Source: CAD feature listing. Evaluate the final solid. Frame: model axes, mm. A direction names the side the tool comes from. Coordinates: 2 decimals unless noted, no trailing zeros. Write each loop counter-clockwise with the first axis right and the second up, starting at its lowest first coordinate (ties: lowest second). Pieces come first, ordered by that corner, then holes. Notation, with made-up numbers: (54, 30) - (73, 30) arc R27 ccw to (73, 51) - close; hole circle Ø11 at (70.25, 13.5). An arc over 180 degrees is marked (long way). One line per question, with ' | ' between items. Start each with the question number.
Q1. Draft query along Y for faces 1 (the face through (71, -23.57, 14.2)), 2 (the face through (-72.15, -56.99, 20.28)), 3 (the face through (0.91, 57.15, 46.99)), 4 (the face through (-18.07, -0.28, 31.5)). Return one class per face: +Y half, -Y half, draft (parallel to the pull), parting line (faces both ways), or undercut.
Q2. Cut plane D-D, the plane y = 23. Return loops of the section in (x, z), plus the area to 3 significant figures.
Q3. Cut plane A-A, the plane y = 0. Return loops of the section in (x, z).
Q4. Cut plane B-B, the plane z = 35.5. Return loops of the section in (x, y), plus the area to 3 significant figures.
Q5. Line query: line 1 (Y direction, x = -43, z = 13.5); line 2 (Y direction, x = 54, z = 27); line 3 (Z direction, x = 37, y = 7). Output: solid intervals per line, ascending.
Q6. Cut plane C-C, the plane x = 5. Return loops of the section in (y, z).
Q7. Contact query for flat-ended pins moving along their axis: P1, Ø0.8, axis at x = 74.5, y = -1.5, coming from the +Z side; P2, Ø20, axis at x = 31, y = 6, coming from the -Z side. Output: stop coordinate, or through.
Q8. Access query for faces 5 (the face through (-72.15, 56.99, 20.28)), 6 (the face through (27, -24, 31)). Directions: +Z, -Z, +X, -X, +Y, -Y. A direction counts if a zero-diameter tool reaches every point of the face in a straight line with its end or side. Return the directions, or none.
```python
from build123d import *

# Parameters (mm, degrees)
F0_W     = 150
F0_H     = 120
F1_DEPTH = 50
F2_R     = 10
F3_W     = 92
F3_H     = 50
F4_DEPTH = 33
F5_R     = 5
F6_W     = 25
F6_H     = 10.0465611815
F7_DEPTH = 40
F9_DEPTH = 25


with BuildPart() as f1:
    # F0 (on Top) → F1 (new body)
    with BuildSketch(Plane.XY):
        Rectangle(F0_W, F0_H)
    extrude(amount=F1_DEPTH)

    # F2
    f2_edges = [f1.edges().sort_by_distance(p)[0] for p in [
        (0, -60, 50),
        (-75, 0, 50),
        (0, 60, 50),
        (75, 0, 50),
        (-75, -60, 25),
        (75, -60, 25),
        (75, 60, 25),
        (-75, 60, 25),
    ]]
    fillet(f2_edges, radius=F2_R)

    # F3 (on face) → F4 (cut)
    with BuildSketch(Plane(origin=(0, 0, 0), x_dir=(1, 0, 0), z_dir=(0, 0, -1))):
        with Locations((26.5, 0)):
            Rectangle(F3_W, F3_H)
    extrude(amount=-F4_DEPTH, mode=Mode.SUBTRACT)

    # F5
    f5_edges = [f1.edges().sort_by_distance(p)[0] for p in [
        (26.5, 25, 33),
        (72.5, 0, 33),
        (26.5, -25, 33),
        (-19.5, 0, 33),
        (-19.5, -25, 16.5),
        (72.5, -25, 16.5),
        (-19.5, 25, 16.5),
        (72.5, 25, 16.5),
    ]]
    fillet(f5_edges, radius=F5_R)

    # F6 (on face) → F7 (cut)
    with BuildSketch(Plane(origin=(0, 0, 0), x_dir=(1, 0, 0), z_dir=(0, 0, -1))):
        with Locations((-32, -14)):
            Rectangle(F6_W, F6_H)
    extrude(amount=-F7_DEPTH, mode=Mode.SUBTRACT)

    # F8 (on face) → F9 (cut)
    with BuildSketch(Plane.YZ.offset(75)):
        with BuildLine():
            Line((12, 18), (0, 18))
            ThreePointArc((0, 18), (1.7573593129, 13.7573593129), (6, 12))
            ThreePointArc((6, 12), (10.2426406871, 13.7573593129), (12, 18))
        make_face()
        with BuildLine():
            ThreePointArc((6, 24), (1.7573593129, 22.2426406871), (0, 18))
            Line((0, 18), (12, 18))
            ThreePointArc((12, 18), (10.2426406871, 22.2426406871), (6, 24))
        make_face()
        with BuildLine():
            ThreePointArc((-6, 24), (-1.7573593129, 22.2426406871), (0, 18))
            ThreePointArc((0, 18), (1.7573593129, 22.2426406871), (6, 24))
            Line((6, 24), (-6, 24))
        make_face()
        with BuildLine():
            Line((-12, 18), (0, 18))
            ThreePointArc((0, 18), (-1.7573593129, 22.2426406871), (-6, 24))
            ThreePointArc((-6, 24), (-10.2426406871, 22.2426406871), (-12, 18))
        make_face()
        with BuildLine():
            ThreePointArc((-6, 12), (-1.7573593129, 13.7573593129), (0, 18))
            Line((0, 18), (-12, 18))
            ThreePointArc((-12, 18), (-10.2426406871, 13.7573593129), (-6, 12))
        make_face()
        with BuildLine():
            ThreePointArc((6, 12), (1.7573593129, 13.7573593129), (0, 18))
            ThreePointArc((0, 18), (-1.7573593129, 13.7573593129), (-6, 12))
            Line((-6, 12), (6, 12))
        make_face()
    extrude(amount=-F9_DEPTH, mode=Mode.SUBTRACT)


solid = f1.part
```
Reply:
1) face 1: undercut | face 2: -Y half | face 3: +Y half | face 4: undercut
2) outline: (-75, 0) - (-18.5, 0) - (-18.5, 28) arc R4 cw to (-14.5, 32) - (67.5, 32) arc R4 cw to (71.5, 28) - (71.5, 0) - (75, 0) - (75, 40) arc R10 ccw to (65, 50) - (-65, 50) arc R10 ccw to (-75, 40) - close | area: 4,580 mm^2
3) outline: (-75, 0) - (-19.5, 0) - (-19.5, 28) arc R5 cw to (-14.5, 33) - (67.5, 33) arc R5 cw to (72.5, 28) - (72.5, 24) - (75, 24) - (75, 40) arc R10 ccw to (65, 50) - (-65, 50) arc R10 ccw to (-75, 40) - close; (72.5, 0) - (75, 0) - (75, 12) - (72.5, 12) - close
4) outline: (-75, -50) arc R10 ccw to (-65, -60) - (65, -60) arc R10 ccw to (75, -50) - (75, 50) arc R10 ccw to (65, 60) - (-65, 60) arc R10 ccw to (-75, 50) - close; hole (-44.5, 8.98) - (-19.5, 8.98) - (-19.5, 19.02) - (-44.5, 19.02) - close | area: 17,700 mm^2
5) line 1: y = -60 to 8.98, 19.02 to 60 | line 2: y = -60 to -25, 25 to 60 | line 3: z = 33 to 50
6) outline: (-60, 0) - (-25, 0) - (-25, 28) arc R5 cw to (-20, 33) - (20, 33) arc R5 cw to (25, 28) - (25, 0) - (60, 0) - (60, 40) arc R10 ccw to (50, 50) - (-50, 50) arc R10 ccw to (-60, 40) - close
7) P1: stops at z = 44.15 | P2: stops at z = 33
8) face 5: +Z, -Z, -X, +Y | face 6: -Z
